Here's the drawing with two shaded views (mm, measured from the low corner). I have some questions. A direction names the side the tool comes from. Coordinates: 2 decimals unless noted, no trailing zeros. Write each loop counter-clockwise with the first axis right and the second up, starting at its lowest first coordinate (ties: lowest second). Pieces come first, ordered by that corner, then holes.
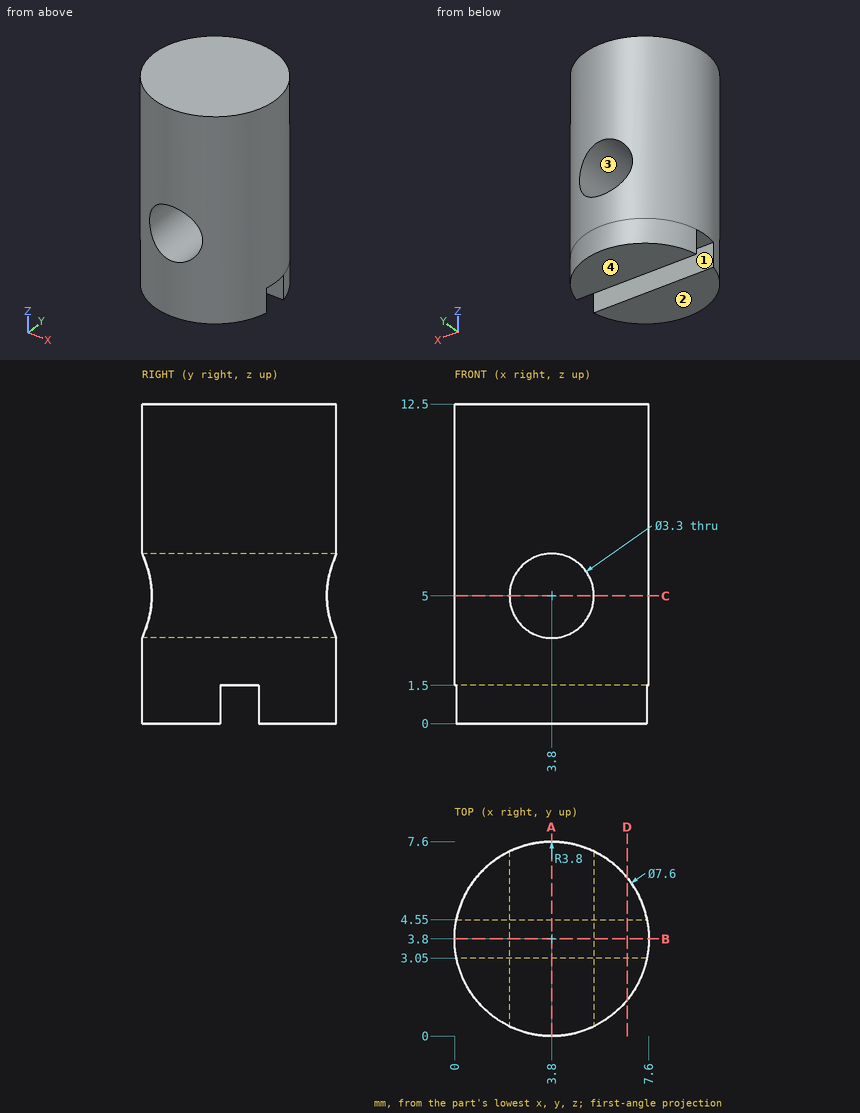
1. If we mould it in two halves opening along X, with no side actions, what happens to the marked faces 3 and 4? For each: pulls with the +X half, pulls with the -X half, needs draft (parallel to the pull), parting line crosses it, or undercut.
Verdict:
face 3: undercut
face 4: needs draft
2. I want a section at C-C on z = 5. Please give me the cut outline in (x, y), plus the area to 3 significant figures.
Verdict:
outline: (2.15, 0.38) - (2.15, 7.22) arc R3.8 ccw to start; (5.45, 0.38) arc R3.8 ccw to (5.45, 7.22) - close
area: 21.1 mm2
3. I want a section at A-A on x = 3.8. Please give me the cut outline in (y, z).
Verdict:
outline: (0, 0) - (3.05, 0) - (3.05, 1.5) - (4.55, 1.5) - (4.55, 0) - (7.6, 0) - (7.6, 3.35) - (0, 3.35) - close; (0, 6.65) - (7.6, 6.65) - (7.6, 12.5) - (0, 12.5) - close
4. Please list where these lines run through material, in increasing order: line 1 along Z through (x, y) = (3.75, 6.5); line 2 along X through (y, z) = (2.5, 5); line 3 along X through (y, z) = (3, 5).
Verdict:
line 1: z = 0 to 3.35, 6.65 to 12.5
line 2: x = 0.23 to 2.15, 5.45 to 7.37
line 3: x = 0.09 to 2.15, 5.45 to 7.51
5. I want a section at D-D on x = 6.75. Please give me the cut outline in (y, z), plus the area to 3 significant figures.
Verdict:
outline: (1.4, 0) - (3.05, 0) - (3.05, 1.5) - (4.55, 1.5) - (4.55, 0) - (6.2, 0) - (6.2, 12.5) - (1.4, 12.5) - close
area: 57.6 mm2
6. On a 3-axis mill with a long thin cutter (end or side, diameter ignored), from which of +Z, -Z, +X, -X, +Y, -Y can I reach the whole of each face in a straight line? I mean the marked faces 1 and 2. Say none if no direction works.
Verdict:
face 1: -Z, +X, -X
face 2: -Z, +X, -X, +Y, -Y
7. For pin 1 (1.2 mm diameter, centred on x = 2.5, y = 4, fed in from -Z); pin 2 (1.5 mm diameter, centred on x = 5, z = 10.5, fed in from -Y); pin 3 (0.8 mm diameter, centred on x = 4.5, z = 1, fed in from +Y); pin 4 (1 mm diameter, centred on x = 7, z = 8, fed in from -Y), each with a flat end and sliding along its axis, tell me the tip position at first contact or that it passes through.
Verdict:
pin 1: stops at z = 0
pin 2: stops at y = 0.03
pin 3: stops at y = 7.59
pin 4: stops at y = 1.13
8. I want a section at B-B on y = 3.8. Please give me the cut outline in (x, z), plus the area to 3 significant figures.
Verdict:
outline: (0, 1.5) - (7.6, 1.5) - (7.6, 12.5) - (0, 12.5) - close; hole circle Ø3.3 at (3.8, 5)
area: 75.0 mm2
